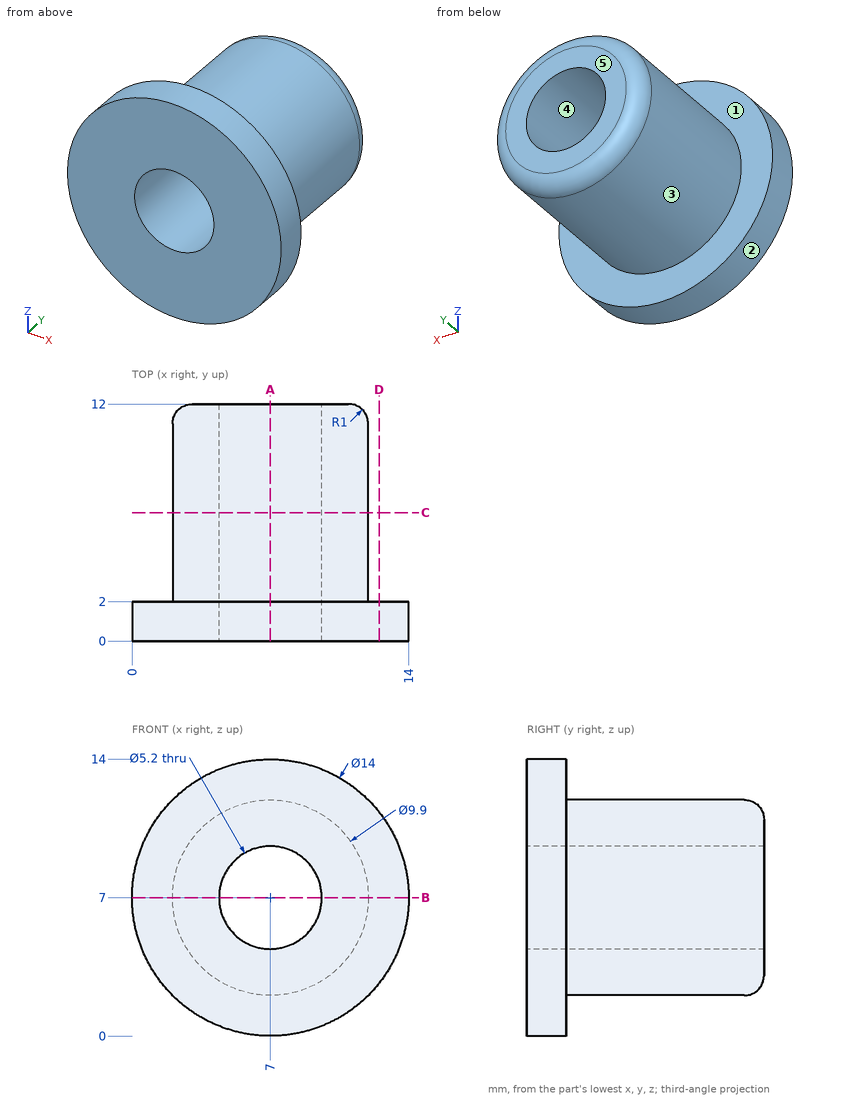
Answer from the drawing. Dimensions are ordinates in mm from the lowest x, y and z of the part. A direction names the side the tool comes from. Round coordinates to 2 decimals unless told otherwise and drop trailing zeros. Write each loop counter-clockwise with the first axis right and the second up, starting at its lowest first coordinate (ties: lowest second). Pieces come first, ordered by that corner, then holes. Notation, with made-up numbers: M 86,73 L 95,73 A27 cw 95,105 Z; hole C 6,-22 d3. An arc over 180 degrees is marked long. One line per item, written item: value.
Q1. Find section A-A on x = 7. Write down the section's boundary in (y, z).
Data:
outline: M 0,0 L 2,0 L 2,2.05 L 11,2.05 A1 ccw 12,3.05 L 12,4.4 L 0,4.4 Z; M 0,9.6 L 12,9.6 L 12,10.95 A1 ccw 11,11.95 L 2,11.95 L 2,14 L 0,14 Z
Q2. Find section D-D on x = 12.5. Write down the section's boundary in (y, z).
Data:
outline: M 0,2.67 L 2,2.67 L 2,11.33 L 0,11.33 Z
Q3. Straight lines are drawn through the part: line 1 (Z direction, x = 7, y = 3.5); line 2 (X direction, y = 1.5, z = 6.5); line 3 (Z direction, x = 5, y = 6.25). For each, find the intervals that lie inside material, in ascending order. Write a range as [from, to].
Data:
line 1: [2.05, 4.4], [9.6, 11.95]
line 2: [0.02, 4.45], [9.55, 13.98]
line 3: [2.47, 5.34], [8.66, 11.53]
Q4. Find section B-B on z = 7. Write down the section's boundary in (x, y), plus the area to 3 significant figures.
Data:
outline: M 0,0 L 4.4,0 L 4.4,12 L 3.05,12 A1 ccw 2.05,11 L 2.05,2 L 0,2 Z; M 9.6,0 L 14,0 L 14,2 L 11.95,2 L 11.95,11 A1 ccw 10.95,12 L 9.6,12 Z
area: 64.2 mm2
Q5. Which of the six approach directions +Z, -Z, +X, -X, +Y, -Y give full straight-line access (tool end or side, diameter ignored) to the marked faces 1 and 2?
Data:
face 1: +Y
face 2: +Y, -Y
Q6. Find section C-C on y = 6.5. Write down the section's boundary in (x, z).
Data:
outline: C 7,7 d9.9; hole C 7,7 d5.2
Q7. Flat-ended cylindrical pins translate along their axes: pin 1 Ø4 at (x, y) = (4, 7.5) entering from +Z; pin 2 Ø3 at (y, z) = (3, 1.5) entering from +X; pin 3 Ø6 at (y, z) = (10.5, 5) entering from +X. Find the tip coordinate at first contact, or state that the pin passes through.
Data:
pin 1: z = 11.85
pin 2: x = 12.46
pin 3: x = 11.95
Q8. For a pull along Z with two mould halves and no side action, classify the marked faces 3, 4 and 5 as +Z half, -Z half, draft (parallel to the pull), parting line (faces both ways), or undercut.
Data:
face 3: parting line
face 4: undercut
face 5: draft
